```python
from build123d import *

# Parameters (mm, degrees)
RESSALTO_EXTRUS_O1_DEPTH = 10
CORTE_EXTRUS_O1_DEPTH    = 10
RESSALTO_EXTRUS_O2_DEPTH = 1
ESBO_O4_R                = 3
RESSALTO_EXTRUS_O3_DEPTH = 5
ESBO_O5_R                = 6
RESSALTO_EXTRUS_O4_DEPTH = 1.7


with BuildPart() as part:
    # Esboço1 → Ressalto-extrusão1 (new, symmetric)
    with BuildSketch(Plane.XY):
        Polygon((20, -0.767915455), (25.568877633, -0.767915455), (25.568877633, -3.767915455), (20, -3.767915455), (20, -30.767915455), (-20, -30.767915455), (-20, -3.767915455), (-25.568877633, -3.767915455), (-25.568877633, -0.767915455), (-20, -0.767915455), (-20, 4.732084545), (20, 4.732084545), align=None)
    extrude(amount=RESSALTO_EXTRUS_O1_DEPTH, both=True)

    # Esboço6 → Corte-extrusão1 (cut)
    with BuildSketch(Plane(origin=(0, -0.767915455, 0), x_dir=(1, 0, 0), z_dir=(0, 1, 0))):
        with BuildLine():
            Line((25.071445053, 4), (25.568877633, 4))
            Line((25.568877633, 4), (25.568877633, 6))
            Line((25.568877633, 6), (25.071445053, 6))
            ThreePointArc((25.071445053, 6), (23.061122367, 5), (25.071445053, 4))
        make_face()
        with BuildLine():
            Line((25.568877633, -6), (25.568877633, -4))
            Line((25.568877633, -4), (25.071445053, -4))
            ThreePointArc((25.071445053, -4), (23.061122367, -5), (25.071445053, -6))
            Line((25.071445053, -6), (25.568877633, -6))
        make_face()
        with BuildLine():
            ThreePointArc((-25.071445053, 6), (-23.061122367, 5), (-25.071445053, 4))
            Line((-25.071445053, 4), (-25.568877633, 4))
            Line((-25.568877633, 4), (-25.568877633, 6))
            Line((-25.568877633, 6), (-25.071445053, 6))
        make_face()
        with BuildLine():
            ThreePointArc((-25.071445053, -4), (-23.061122367, -5), (-25.071445053, -6))
            Line((-25.071445053, -6), (-25.568877633, -6))
            Line((-25.568877633, -6), (-25.568877633, -4))
            Line((-25.568877633, -4), (-25.071445053, -4))
        make_face()
    extrude(amount=-CORTE_EXTRUS_O1_DEPTH, mode=Mode.SUBTRACT)

    # Esboço3 → Ressalto-extrusão2 (add)
    with BuildSketch(Plane(origin=(0, 4.732084545, 0), x_dir=(1, 0, 0), z_dir=(0, 1, 0))):
        with BuildLine():
            Line((-19, 9.202511885), (10.015, 9.202511885))
            ThreePointArc((10.015, 9.202511885), (19.216883893, -0.107507336), (9.8, -9.2))
            Line((9.8, -9.2), (-19, -9.2))
            Line((-19, -9.2), (-19, 9.202511885))
        make_face()
    extrude(amount=RESSALTO_EXTRUS_O2_DEPTH)

    # Esboço4 → Ressalto-extrusão3 (add)
    with BuildSketch(Plane(origin=(0, 5.732084545, 0), x_dir=(1, 0, 0), z_dir=(0, 1, 0))):
        with Locations(Location((10.015, 0, 0), (0, 0, 180))):
            Circle(ESBO_O4_R)
    extrude(amount=RESSALTO_EXTRUS_O3_DEPTH)

    # Esboço5 → Ressalto-extrusão4 (add)
    with BuildSketch(Plane(origin=(0, 5.732084545, 0), x_dir=(1, 0, 0), z_dir=(0, 1, 0))):
        with Locations(Location((10.015, 0, 0), (0, 0, 180))):
            Circle(ESBO_O5_R)
    extrude(amount=RESSALTO_EXTRUS_O4_DEPTH)


solid = part.part
```
CAD build for the part. Positions are in the model's coordinates, mm. A direction names the side the tool comes from. Round coordinates to 2 decimals unless told otherwise and drop trailing zeros. Loops run counter-clockwise (first coordinate to the right, second up) from the corner with the lowest first, then second, coordinate; pieces in that order, holes last. Notation, with made-up numbers: M -25.5,84.5 L -9.5,84.5 A35 cw -9.5,117.5 Z; hole C 2,10.25 d8. An arc over 180 degrees is marked long. Use a Markdown table: item, result. Add a question column.
(1) Flat gauge pins, fed straight in: pin 1 (6 mm diameter, centred on x = -21.5, z = -3, fed in from +Y); pin 2 (6 mm diameter, centred on y = -12, z = -3.5, fed in from +X); pin 3 (4.5 mm diameter, centred on x = -23.5, z = -3, fed in from -Y). Where does each tip first touch, or does it go through?
(2) Cut at A-A (x = -14). Give the cut face in (y, z), and give its area (3 significant figures).
(3) Which spindle directions (+Z, -Z, +X, -X, +Y, -Y) get a long thin tool onto all of the face, cutting with end or side? Do faces 5 (the face through (2.9, 4.732, -9.6)), 6 (the face through (-20, 2, 0)), 7 (the face through (-23, -3.768, 0)), 8 (the face through (23, -3.768, 0)). Say none if no direction does.
(4) Pull direction X, two halves, no side cores. Call faces 1 (the face through (23.06, -2.25, 4.96)), 2 (the face through (20, -17, 0)), 3 (the face through (-23.06, -2.25, -5.04)), 4 (the face through (-23, -0.768, 0)): +X half, -X half, draft (parallel to the pull), parting line (faces both ways), or undercut.
(5) Drill centre lines: line 1 (X direction, y = -5.5, z = 1.75); line 2 (Y direction, x = -6.5, z = 6.75); line 3 (Y direction, x = -23, z = 0). Where is each one in solid material? Low to high.
(6) Cut at B-B (z = 0). Give the cut face in (x, y) (3 decimals), and give its area (3 significant figures).
(7) Cut at D-D (z = -7.25). Give the cut face in (x, y), and give its area (3 significant figures).
(8) Cut at C-C (y = -19). Give the cut face in (x, z).
Geometry says:
| question | item | result |
|---|---|---|
| 1 | pin 1 | stops at y = 5.73 |
| 1 | pin 2 | stops at x = 20 |
| 1 | pin 3 | stops at y = -3.77 |
| 2 | outline | M -30.77,-10 L 4.73,-10 L 4.73,-9.2 L 5.73,-9.2 L 5.73,9.2 L 4.73,9.2 L 4.73,10 L -30.77,10 Z |
| 2 | area | 728 mm² |
| 3 | face 5 | +Y |
| 3 | face 6 | +Z, -Z, -X, +Y |
| 3 | face 7 | +Z, -Z, -X, -Y |
| 3 | face 8 | +Z, -Z, +X, -Y |
| 4 | face 1 | undercut |
| 4 | face 2 | +X half |
| 4 | face 3 | undercut |
| 4 | face 4 | draft |
| 5 | line 1 | x = -20 to 20 |
| 5 | line 2 | y = -30.77 to 5.73 |
| 5 | line 3 | y = -3.77 to -0.77 |
| 6 | outline | M -25.569,-3.768 L -20,-3.768 L -20,-30.768 L 20,-30.768 L 20,-3.768 L 25.569,-3.768 L 25.569,-0.768 L 20,-0.768 L 20,4.732 L 19.218,4.732 L 19.218,5.732 L 16.015,5.732 L 16.015,7.432 L 13.015,7.432 L 13.015,10.732 L 7.015,10.732 L 7.015,7.432 L 4.015,7.432 L 4.015,5.732 L -19,5.732 L -19,4.732 L -20,4.732 L -20,-0.768 L -25.569,-0.768 Z |
| 6 | area | 1,530 mm² |
| 7 | outline | M -25.57,-3.77 L -20,-3.77 L -20,-30.77 L 20,-30.77 L 20,-3.77 L 25.57,-3.77 L 25.57,-0.77 L 20,-0.77 L 20,4.73 L 15.68,4.73 L 15.68,5.73 L -19,5.73 L -19,4.73 L -20,4.73 L -20,-0.77 L -25.57,-0.77 Z |
| 7 | area | 1,490 mm² |
| 8 | outline | M -20,-10 L 20,-10 L 20,10 L -20,10 Z |
